Here's how the part is built. I have some questions about the finished solid (model axes, mm). Face numbers are marked on the shaded views. Round coordinates to 2 decimals unless told otherwise and drop trailing zeros. Write each loop counter-clockwise with the first axis right and the second up, starting at its lowest first coordinate (ties: lowest second). Pieces come first, ordered by that corner, then holes. Notation, with made-up numbers: (45.5, 71) -> (86.5, 71) arc R24 cw to (86.5, 108) -> close; hole circle Ø11 at (21, -3.75). An arc over 180 degrees is marked (long way). Answer as CSV lines item,"result".
from build123d import *

# Parameters (mm, degrees)
SKETCH2_R           = 3.5
BOSS_EXTRUDE1_DEPTH = 21
SKETCH7_R           = 1.05
CUT_EXTRUDE2_DEPTH  = 6
SKETCH4_W           = 4.65
SKETCH4_H           = 4.65
CUT_EXTRUDE5_DEPTH  = 10.2


with BuildPart() as part:
    # Sketch2 → Boss-Extrude1 (new body)
    with BuildSketch(Plane.XY):
        with Locations(Location((0, 0, 0), (0, 0, 180))):
            Circle(SKETCH2_R)
    extrude(amount=BOSS_EXTRUDE1_DEPTH)

    # Sketch7 → Cut-Extrude2 (cut)
    with BuildSketch(Plane.XY.offset(21)):
        Circle(SKETCH7_R)
    extrude(amount=-CUT_EXTRUDE2_DEPTH, mode=Mode.SUBTRACT)

    # Sketch4 → Cut-Extrude5 (cut)
    with BuildSketch(Plane(origin=(0, 0, 0), x_dir=(-1, 0, 0), z_dir=(0, 0, -1))):
        Rectangle(SKETCH4_W, SKETCH4_H)
    extrude(amount=-CUT_EXTRUDE5_DEPTH, mode=Mode.SUBTRACT)


solid = part.part
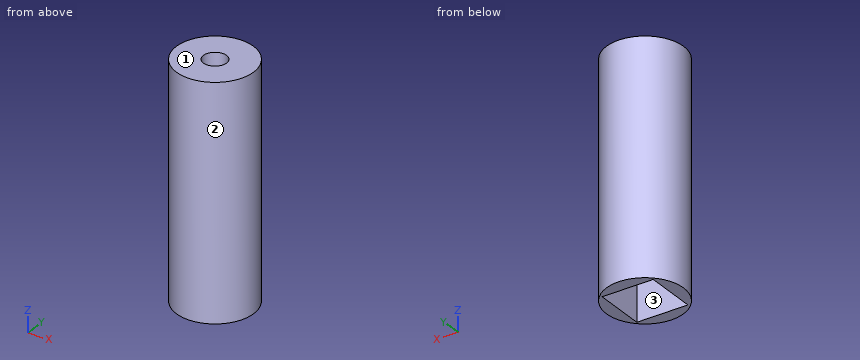
Item 1: Suppose I cut it at D-D, the plane y = -1.5. List the corners of the cut face in (x, z) for me (3 decimals).
Results found:
outline,"(-3.162, 0) -> (-2.325, 0) -> (-2.325, 10.2) -> (2.325, 10.2) -> (2.325, 0) -> (3.162, 0) -> (3.162, 21) -> (-3.162, 21) -> close"
Item 2: Suppose I cut it at B-B, the plane z = 6. List the corners of the cut face in (x, y) for me (3 decimals), then the cut area to 3 significant figures.
Results found:
outline,"circle Ø7 at (0, 0); hole (-2.325, -2.325) -> (2.325, -2.325) -> (2.325, 2.325) -> (-2.325, 2.325) -> close"
area,"16.9 mm²"
Item 3: Will these pins go through, and if not, where does the flat tip stop? pin 1 (2 mm diameter, centred on y = -0.5, z = 17, fed in from +X); pin 2 (2.5 mm diameter, centred on x = -0.5, y = 0.5, fed in from -Z); pin 3 (1.5 mm diameter, centred on y = -2.5, z = 12, fed in from +X); pin 4 (1.3 mm diameter, centred on x = 0, y = 0, fed in from +Z).
Results found:
pin 1,"stops at x = 3.5"
pin 2,"stops at z = 10.2"
pin 3,"stops at x = 3.03"
pin 4,"stops at z = 15"
Item 4: If we mould it in two halves opening along Y, with no side actions, what happens to the marked faces 1, 2 and 3? For each: pulls with the +Y half, pulls with the -Y half, needs draft (parallel to the pull), parting line crosses it, or undercut.
Results found:
face 1,"needs draft"
face 2,"parting line crosses it"
face 3,"undercut"
Item 5: Suppose I cut it at A-A, the plane y = 0. List the corners of the cut face in (x, z) for me (3 decimals).
Results found:
outline,"(-3.5, 0) -> (-2.325, 0) -> (-2.325, 10.2) -> (2.325, 10.2) -> (2.325, 0) -> (3.5, 0) -> (3.5, 21) -> (1.05, 21) -> (1.05, 15) -> (-1.05, 15) -> (-1.05, 21) -> (-3.5, 21) -> close"
Item 6: I need wall thicknesses on L1, parallel to Y at x = 0, z = 18.4; L2, parallel to Y at x = 0.75, z = 2.5 (3 decimals); L3, parallel to X at y = 0.25, z = 2.75 (3 decimals). Which ranges of each line are inside material? Lowest first, please.
Results found:
L1,"y = -3.5 to -1.05, 1.05 to 3.5"
L2,"y = -3.419 to -2.325, 2.325 to 3.419"
L3,"x = -3.491 to -2.325, 2.325 to 3.491"
